Could you check a few things on this model? Use its own coordinates, in mm. A direction names the side the tool comes from. Coordinates: 2 decimals unless noted, no trailing zeros. Loops run counter-clockwise (first coordinate to the right, second up) from the corner with the lowest first, then second, coordinate; pieces in that order, holes last.
from build123d import *

# Parameters (mm, degrees)
SKETCH2_R          = 3.75
CUT_EXTRUDE1_DEPTH = 10


with BuildPart() as part:
    # Sketch1 → Revolve1 (revolve)
    with BuildSketch(Plane.XY, mode=Mode.PRIVATE) as revolve1_sk:
        Polygon((0, 1.5), (0, 19.5), (1, 19.5), (1, 20), (1.5, 20), (1.5, 25), (-7, 25), (-7, 20), (-6.5, 20), (-6.5, 19.5), (-3.175, 19.5), (-3.175, 5), (-7, 5), (-7, 1.5), (-3.175, 1.5), align=None)
    revolve(revolve1_sk.sketch.rotate(Axis((-3.175, 0, 0), (1, 0, 0)), 90), axis=Axis((-3.175, 0, 0), (1, 0, 0)))

    # Sketch2 → Cut-Extrude1 (cut)
    with BuildSketch(Plane.ZY.offset(3.175)):
        with Locations((0, 12)):
            Circle(SKETCH2_R)
        with Locations((10.392304845, 6)):
            Circle(SKETCH2_R)
        with Locations((10.392304845, -6)):
            Circle(SKETCH2_R)
        with Locations((0, -12)):
            Circle(SKETCH2_R)
        with Locations((-10.392304845, -6)):
            Circle(SKETCH2_R)
        with Locations((-10.392304845, 6)):
            Circle(SKETCH2_R)
    extrude(amount=-CUT_EXTRUDE1_DEPTH, mode=Mode.SUBTRACT)


solid = part.part
(1) Imagine slicing it at B-B, the plane z = 0. State how many separate pieces and enclosed holes the cut face has, and give its area (3 significant figures).
Answers:
separate pieces: 4
enclosed holes: 0
area: 186 mm2
(2) We'd pull the mould along Y, two halves only. Please class faces 4 (the face through (1.5, -17, 11)), 5 (the face through (-1.61, -8.282, -0.488)): +Y half, -Y half, draft (parallel to the pull), parting line (faces both ways), or undercut.
Answers:
face 4: draft
face 5: undercut
(3) Which directions (+Z, -Z, +X, -X, +Y, -Y) give clear straight access to the entire face, cutting with the end or side of a thin tool? Please do faces 1 (the face through (-4.814, -19.334, -2.539)), 2 (the face through (1, 4.4, -19.2)), 3 (the face through (-1.61, 3.72, -13.37)).
Answers:
face 1: -X
face 2: +X
face 3: +X, -X
(4) I need wall thicknesses on probe 1 along Y at (x, z) = (-6.65, 0); probe 2 along Y at (x, z) = (-4.05, 0); probe 3 along Y at (x, z) = (1.4, 0). Which ranges of each line are inside material? Lowest first, please.
Answers:
probe 1: y = -25 to -20, -5 to -1.5, 1.5 to 5, 20 to 25
probe 2: y = -25 to -19.5, -5 to -1.5, 1.5 to 5, 19.5 to 25
probe 3: y = -25 to -20, 20 to 25
(5) Imagine slicing it at C-C, the plane y = -6. Write out the boundary of the cut face in (x, z) (3 decimals).
Answers:
outline: (-7, -24.269) - (1.5, -24.269) - (1.5, -19.079) - (1, -19.079) - (1, -18.554) - (0, -18.554) - (0, -14.142) - (-3.175, -14.142) - (-3.175, -18.554) - (-6.5, -18.554) - (-6.5, -19.079) - (-7, -19.079) - close; (-7, 19.079) - (-6.5, 19.079) - (-6.5, 18.554) - (-3.175, 18.554) - (-3.175, 14.142) - (0, 14.142) - (0, 18.554) - (1, 18.554) - (1, 19.079) - (1.5, 19.079) - (1.5, 24.269) - (-7, 24.269) - close; (-3.175, -6.642) - (0, -6.642) - (0, 6.642) - (-3.175, 6.642) - close
(6) Imagine slicing it at D-D, the plane z = 17.5. Write out the boundary of the cut face in (x, y) (3 decimals).
Answers:
outline: (-7, -17.854) - (1.5, -17.854) - (1.5, -9.682) - (1, -9.682) - (1, -8.602) - (0, -8.602) - (0, 8.602) - (1, 8.602) - (1, 9.682) - (1.5, 9.682) - (1.5, 17.854) - (-7, 17.854) - (-7, 9.682) - (-6.5, 9.682) - (-6.5, 8.602) - (-3.175, 8.602) - (-3.175, -8.602) - (-6.5, -8.602) - (-6.5, -9.682) - (-7, -9.682) - close
(7) Imagine slicing it at A-A, the plane y = 0. Write out the boundary of the cut face in (x, z) (3 decimals), and give its area (3 significant figures).
Answers:
outline: (-7, -25) - (1.5, -25) - (1.5, -20) - (1, -20) - (1, -19.5) - (0, -19.5) - (0, -1.5) - (-7, -1.5) - (-7, -5) - (-3.175, -5) - (-3.175, -19.5) - (-6.5, -19.5) - (-6.5, -20) - (-7, -20) - close; (-7, 1.5) - (0, 1.5) - (0, 19.5) - (1, 19.5) - (1, 20) - (1.5, 20) - (1.5, 25) - (-7, 25) - (-7, 20) - (-6.5, 20) - (-6.5, 19.5) - (-3.175, 19.5) - (-3.175, 5) - (-7, 5) - close
area: 234 mm2
(8) For pin 1 (5 mm diameter, centred on x = -1.5, z = 0, fed in from -Y); pin 2 (5 mm diameter, centred on x = -1.5, z = -9.5, fed in from +Y); pin 3 (10 mm diameter, centred on y = -6, z = -10.39, fed in from -X) (3 decimals), each with a flat end and sliding along its axis, tell me the tip position at first contact or that it passes through.
Answers:
pin 1: stops at y = -25
pin 2: stops at y = 24
pin 3: stops at x = -3.175
